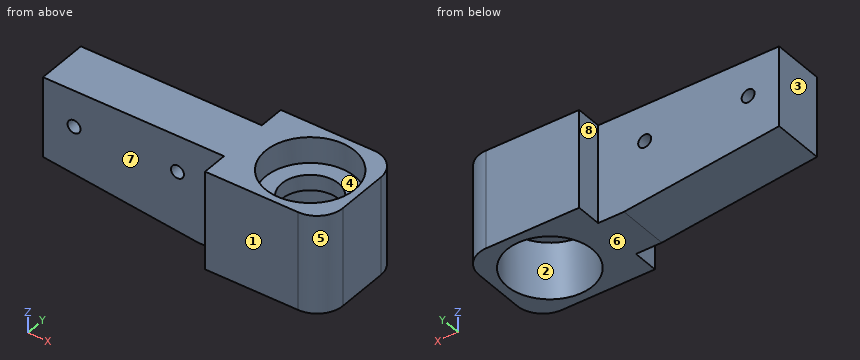
```python
from build123d import *

# Parameters (mm, degrees)
F1_DEPTH       = 20
F3_D           = 11
F3_CBORE_D     = 17.25
F3_CBORE_DEPTH = 5
F4_R           = 8.25
F5_DEPTH       = 11
F7_DEPTH       = 5
F9_DEPTH       = 5
F11_D          = 2.5
F12_R          = 5


with BuildPart() as f1:
    # F0 (on Front) → F1 (new body)
    with BuildSketch(Plane.XZ):
        Polygon((58, 0), (0, 0), (0, -15.5), (30, -19), (58, -19), align=None)
    extrude(amount=F1_DEPTH)

    # F3 (through all)
    with Locations(Plane.XY):
        with Locations((48, -10)):
            CounterBoreHole(F3_D / 2, F3_CBORE_D / 2, F3_CBORE_DEPTH)

    # F4 (on face) → F5 (cut)
    with BuildSketch(Plane(origin=(0, 0, -19), x_dir=(1, 0, 0), z_dir=(0, 0, -1))):
        with Locations((48, 10)):
            Circle(F4_R)
    extrude(amount=-F5_DEPTH, mode=Mode.SUBTRACT)

    # F6 (on face) → F7 (cut)
    with BuildSketch(Plane.XZ.offset(20)):
        Polygon((35, -19), (35, 0), (0, 0), (0, -15.5), (30, -19), align=None)
    extrude(amount=-F7_DEPTH, mode=Mode.SUBTRACT)

    # F8 (on face) → F9 (cut)
    with BuildSketch(Plane(origin=(0, 0, 0), x_dir=(-1, 0, 0), z_dir=(0, 1, 0))):
        Polygon((0, 0), (-35, 0), (-35, -19), (-30, -19), (0, -15.5), align=None)
    extrude(amount=-F9_DEPTH, mode=Mode.SUBTRACT)

    # F11 (through all)
    with Locations(Plane.XZ.offset(15)):
        with Locations((6, -7), (26, -7)):
            Hole(F11_D / 2)

    # F12
    f12_edges = [f1.edges().sort_by_distance(p)[0] for p in [
        (58, -20, -9.5),
        (58, 0, -9.5),
    ]]
    fillet(f12_edges, radius=F12_R)


solid = f1.part
```
Geometry check sheet. Reference: the model listing, model coordinates, mm. Face numbers are marked on the shaded views. A direction names the side the tool comes from. Coordinates: 2 decimals unless noted, no trailing zeros. Loops run counter-clockwise (first coordinate to the right, second up) from the corner with the lowest first, then second, coordinate; pieces in that order, holes last.
Item 1: Release check for a two-part mould opening along Y. For the marked faces 1, 2 and 3 record: released by +Y, released by -Y, zero draft, split by the parting line, or undercut.
Item 2: Access from +Z, -Z, +X, -X, +Y, -Y to the whole of each face (thin tool, end or side, straight path). Record for the marked faces 4, 5, 6, 7 and 8.
Item 3: Go/stop test with flat-tipped pins: pin 1 Ø5.5 at (x, z) = (14.5, -6) entering from +Y; pin 2 Ø6.5 at (x, y) = (48, -10) entering from -Z; pin 3 Ø10 at (y, z) = (-17, -2) entering from +X; pin 4 Ø3 at (x, y) = (50.5, -3.5) entering from +Z. Record where each tip stops, or that it passes through.
Item 4: Sectioned sample at A-A, the plane z = -7. Record the boundary of the cut face in (x, y), then the cut area to 3 significant figures.
Item 5: Sectioned sample at C-C, the plane x = 48. Record the boundary of the cut face in (y, z) (3 decimals), then the cut area to 4 significant figures.
Item 6: Sectioned sample at B-B, the plane y = -8. Record the boundary of the cut face in (x, z).
Item 7: Sectioned sample at D-D, the plane z = -10. Record the boundary of the cut face in (x, y).
Item 8: Thickness scan on line 1 (Y direction, x = 48, z = -11.25); line 2 (Y direction, x = 48, z = -6.85); line 3 (X direction, y = -10, z = -11.5). Record the ranges inside material, lowest first.
Check result:
1. face 1: released by -Y
1. face 2: undercut
1. face 3: zero draft
2. face 4: +Z
2. face 5: +Z, -Z, +X, -Y
2. face 6: -Z, +X, -X, +Y, -Y
2. face 7: +Z, -Z, -X, -Y
2. face 8: +Z, -Z, -X, +Y
3. pin 1: stops at y = -5
3. pin 2: passes through
3. pin 3: stops at x = 58
3. pin 4: stops at z = -5
4. outline: (0, -15) - (4.75, -15) - (4.75, -5) - (0, -5) - close; (7.25, -15) - (24.75, -15) - (24.75, -5) - (7.25, -5) - close; (27.25, -15) - (35, -15) - (35, -20) - (53, -20) arc R5 ccw to (58, -15) - (58, -5) arc R5 ccw to (53, 0) - (35, 0) - (35, -5) - (27.25, -5) - close; hole circle Ø11 at (48, -10)
4. area: 654 mm2
5. outline: (-20, -19) - (-18.25, -19) - (-18.25, -8) - (-15.5, -8) - (-15.5, -5) - (-18.625, -5) - (-18.625, 0) - (-20, 0) - close; (-4.5, -8) - (-1.75, -8) - (-1.75, -19) - (0, -19) - (0, 0) - (-1.375, 0) - (-1.375, -5) - (-4.5, -5) - close
5. area: 79.25 mm2
6. outline: (0, -15.5) - (30, -19) - (40, -19) - (40, -8) - (42.88, -8) - (42.88, -5) - (39.61, -5) - (39.61, 0) - (0, 0) - close; (53.12, -8) - (56, -8) - (56, -19) - (58, -19) - (58, 0) - (56.39, 0) - (56.39, -5) - (53.12, -5) - close; hole circle Ø2.5 at (6, -7); hole circle Ø2.5 at (26, -7)
7. outline: (0, -15) - (35, -15) - (35, -20) - (53, -20) arc R5 ccw to (58, -15) - (58, -5) arc R5 ccw to (53, 0) - (35, 0) - (35, -5) - (0, -5) - close; hole circle Ø16.5 at (48, -10)
8. line 1: y = -20 to -18.25, -1.75 to 0
8. line 2: y = -20 to -15.5, -4.5 to 0
8. line 3: x = 0 to 39.75, 56.25 to 58
